```python
from build123d import *

# Parameters (mm, degrees)
SKETCH_1_W      = 37.5
SKETCH_1_H      = 33.5
SKETCH_1_R      = 3
SKETCH_1_R_2    = 1
EXTRUDE_1_DEPTH = 3
SKETCH_1_3_R    = 12
SKETCH_1_3_R_2  = 11.5
EXTRUDE_2_DEPTH = 10.5
FILLET_1_R      = 3


with BuildPart() as part:
    # Sketch 1 → Extrude 1 (new body)
    with BuildSketch(Plane(origin=(0, 0, 0), x_dir=(1, 0, 0), z_dir=(0, 1, 0))):
        Rectangle(SKETCH_1_W, SKETCH_1_H)
        with Locations(Location((-4.25, 0, 0), (0, 0, 270))):
            Circle(SKETCH_1_R, mode=Mode.SUBTRACT)
        with Locations(Location((-11.75, 0, 0), (0, 0, 270))):
            Circle(SKETCH_1_R_2, mode=Mode.SUBTRACT)
        with Locations(Location((-4.25, 7.5, 0), (0, 0, 270))):
            Circle(SKETCH_1_R_2, mode=Mode.SUBTRACT)
        with Locations(Location((3.25, 0, 0), (0, 0, 270))):
            Circle(SKETCH_1_R_2, mode=Mode.SUBTRACT)
        with Locations(Location((-4.25, -7.5, 0), (0, 0, 270))):
            Circle(SKETCH_1_R_2, mode=Mode.SUBTRACT)
        with Locations(Location((-16.25, 14.25, 0), (0, 0, 270))):
            Circle(SKETCH_1_R_2, mode=Mode.SUBTRACT)
        with Locations(Location((-16.25, -14.25, 0), (0, 0, 90))):
            Circle(SKETCH_1_R_2, mode=Mode.SUBTRACT)
        with Locations(Location((16.25, 14.25, 0), (0, 0, 90))):
            Circle(SKETCH_1_R_2, mode=Mode.SUBTRACT)
        with Locations(Location((16.25, -14.25, 0), (0, 0, 270))):
            Circle(SKETCH_1_R_2, mode=Mode.SUBTRACT)
    extrude(amount=EXTRUDE_1_DEPTH)

    # Sketch 1_3 → Extrude 2 (add)
    with BuildSketch(Plane(origin=(0, 0, 0), x_dir=(1, 0, 0), z_dir=(0, 1, 0))):
        with Locations(Location((-4.25, 0, 0), (0, 0, 90))):
            Circle(SKETCH_1_3_R)
        with Locations(Location((-4.25, 0, 0), (0, 0, 90))):
            Circle(SKETCH_1_3_R_2, mode=Mode.SUBTRACT)
    extrude(amount=EXTRUDE_2_DEPTH)

    # Fillet 1
    fillet_1_edges = [part.edges().sort_by_distance(p)[0] for p in [
        (-18.75, 1.5, -16.75),
        (18.75, 1.5, -16.75),
        (18.75, 1.5, 16.75),
        (-18.75, 1.5, 16.75),
    ]]
    fillet(fillet_1_edges, radius=FILLET_1_R)


solid = part.part
```
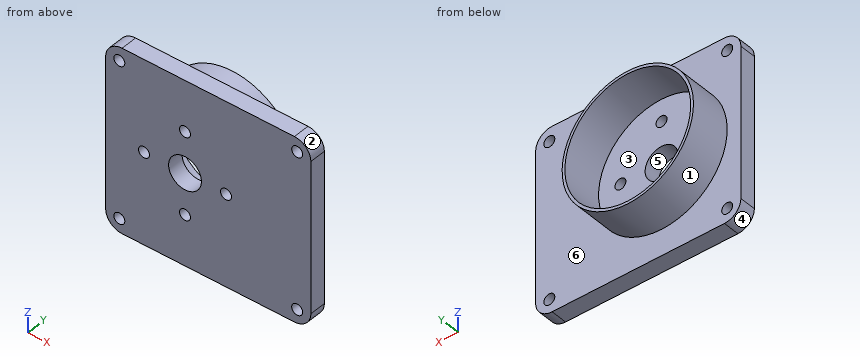
Check sheet for the modelled part. Datum: model origin and axes. Units: mm. Face numbers are marked on the shaded views. A direction names the side the tool comes from. Give positions to 0.01 mm unless a question says otherwise; leave off trailing zeros. Write each loop counter-clockwise with the first axis right and the second up, starting at its lowest first coordinate (ties: lowest second). Pieces come first, ordered by that corner, then holes.
Item 1: Scan lines: L1, parallel to X at y = 1.7, z = 0; L2, parallel to X at y = 1.8, z = 14.25; L3, parallel to Y at x = 2, z = 9. Record each from-to range of solid material in increasing order.
Item 2: Gauge pin test, flat ends, axial feed: pin 1 (2 mm diameter, centred on y = 9, z = 2.5, fed in from +X); pin 2 (6 mm diameter, centred on x = -13.5, z = -11, fed in from -Y); pin 3 (1.2 mm diameter, centred on x = 16.25, z = -14.25, fed in from +Y); pin 4 (2.5 mm diameter, centred on x = 16.25, z = 14.25, fed in from +Y). Record the tip position at first contact, or that the pin passes through.
Item 3: Cross-section at D-D (x = -11.75). Enter the section's corners in (y, z).
Item 4: Access from +Z, -Z, +X, -X, +Y, -Y to the whole of each face (thin tool, end or side, straight path). Record for the marked faces 5 and 6.
Item 5: Draft check along Z on the marked faces 1, 2, 3 and 4. Enter one of: released by +Z, released by -Z, zero draft, split by the parting line, or undercut.
Item 6: Cross-section at C-C (y = 2.5). Count the separate pieces of the cut face and the enclosed holes in it, and give its area (3 significant figures).
Item 7: Cross-section at B-B (z = 0). Enter the section's corners in (x, y).
Item 8: Cross-section at A-A (x = -4.25). Enter the section's corners in (y, z), and give its area (3 significant figures).
Report:
1. L1: x = -18.75 to -12.75, -10.75 to -7.25, -1.25 to 2.25, 4.25 to 18.75
1. L2: x = -18.71 to -17.25, -15.25 to 15.25, 17.25 to 18.71
1. L3: y = 0 to 3
2. pin 1: stops at x = 7.66
2. pin 2: stops at y = 0
2. pin 3: passes through
2. pin 4: stops at y = 3
3. outline: (0, -16.75) - (3, -16.75) - (3, -9.37) - (10.5, -9.37) - (10.5, -8.72) - (3, -8.72) - (3, -1) - (0, -1) - close; (0, 1) - (3, 1) - (3, 8.72) - (10.5, 8.72) - (10.5, 9.37) - (3, 9.37) - (3, 16.75) - (0, 16.75) - close
4. face 5: +Y, -Y
4. face 6: +Y
5. face 1: split by the parting line
5. face 2: released by +Z
5. face 3: undercut
5. face 4: released by -Z
6. separate pieces: 1
6. enclosed holes: 9
6. area: 1,200 mm2
7. outline: (-18.75, 0) - (-12.75, 0) - (-12.75, 3) - (-15.75, 3) - (-15.75, 10.5) - (-16.25, 10.5) - (-16.25, 3) - (-18.75, 3) - close; (-10.75, 0) - (-7.25, 0) - (-7.25, 3) - (-10.75, 3) - close; (-1.25, 0) - (2.25, 0) - (2.25, 3) - (-1.25, 3) - close; (4.25, 0) - (18.75, 0) - (18.75, 3) - (7.75, 3) - (7.75, 10.5) - (7.25, 10.5) - (7.25, 3) - (4.25, 3) - close
8. outline: (0, -16.75) - (3, -16.75) - (3, -12) - (10.5, -12) - (10.5, -11.5) - (3, -11.5) - (3, -8.5) - (0, -8.5) - close; (0, -6.5) - (3, -6.5) - (3, -3) - (0, -3) - close; (0, 3) - (3, 3) - (3, 6.5) - (0, 6.5) - close; (0, 8.5) - (3, 8.5) - (3, 11.5) - (10.5, 11.5) - (10.5, 12) - (3, 12) - (3, 16.75) - (0, 16.75) - close
8. area: 78.0 mm2
